CAD build for the part. Positions are in the model's coordinates, mm. Coordinates: 2 decimals unless noted, no trailing zeros. Write each loop counter-clockwise with the first axis right and the second up, starting at its lowest first coordinate (ties: lowest second). Pieces come first, ordered by that corner, then holes. Notation, with made-up numbers: (31, 73.5) - (65, 73.5) arc R15 ccw to (65, 99.5) - close; hole circle Ø4 at (69, 43.5). An arc over 180 degrees is marked (long way). One line per question, with ' | ' between items. Start each with the question number.
1. Two-plate mould, pull along Z, no slides. Class faces 1 (the flat face through (-33, 5, 10)), 2 (the cylindrical face through (-37.043, 2.465, 3.148)): +Z half, -Z half, draft (parallel to the pull), parting line (faces both ways), or undercut.
2. Flat gauge pins, fed straight in: P1, Ø4.5, axis at x = 27.21, z = -29.32, coming from the +Y side; P2, Ø6.5, axis at x = -39.89, z = 2.99, coming from the -Y side; P3, Ø1, axis at y = 0.5, z = -29.5, coming from the -X side; P4, Ø2, axis at y = 3.5, z = 12, coming from the +X side (3 decimals). Where does each tip first touch, or does it go through?
3. Band-saw the part on C-C, the plane z = -20. Write the cut outline in (x, y).
4. Band-saw the part on D-D, the plane y = 1.25. Give the number of separate pieces and of enclosed holes in the cut face, then the cut area to 3 significant figures.
5. Probe line 1 (X direction, y = 4, z = 0.5); line 2 (Z direction, x = -17, y = 2.95); line 3 (Z direction, x = 25, y = 1.3). List the from-to ranges inside material, lowest first.
6. Band-saw the part on A-A, the plane x = 0. Write the cut outline in (y, z).
7. Band-saw the part on B-B, the plane z = -46. Write the cut outline in (x, y).
from build123d import *

# Parameters (mm, degrees)
SKIZZE1_R                        = 50
SKIZZE1_R_2                      = 33.5
AUFSATZ_LINEAR_AUSTRAGEN1_DEPTH  = 5
F_3_2_3_2_DURCHMESSER_BOHRUNG2_D = 3.2
KREISMUSTER1_COUNT               = 7
F_5_6_5_6_DURCHMESSER_BOHRUNG2_D = 5.7
KREISMUSTER2_COUNT               = 21


with BuildPart() as part:
    # Skizze1 → Aufsatz-Linear austragen1 (new body)
    with BuildSketch(Plane(origin=(0, 0, 0), x_dir=(1, 0, 0), z_dir=(0, 1, 0))):
        with Locations(Location((0, 0, 0), (0, 0, 270))):
            Circle(SKIZZE1_R)
        with Locations(Location((0, 0, 0), (0, 0, 270))):
            Circle(SKIZZE1_R_2, mode=Mode.SUBTRACT)
    extrude(amount=AUFSATZ_LINEAR_AUSTRAGEN1_DEPTH)

    # Ø3.2 (3.2) Durchmesser Bohrung2 (through all)
    with Locations(Plane(origin=(0, 5, 0), x_dir=(1, 0, 0), z_dir=(0, 1, 0))):
        with Locations((0, 46)):
            f_3_2_3_2_durchmesser_bohrung2 = Hole(F_3_2_3_2_DURCHMESSER_BOHRUNG2_D / 2)

    # Kreismuster1: Ø3.2 (3.2) Durchmesser Bohrung2 ×7 about axis
    kreismuster1_axis = Axis((0, 0, 0), (0, 1, 0))
    for i in range(1, KREISMUSTER1_COUNT):
        add(f_3_2_3_2_durchmesser_bohrung2.rotate(kreismuster1_axis, i * 360 / KREISMUSTER1_COUNT), mode=Mode.SUBTRACT)

    # Ø5.6 (5.6) Durchmesser Bohrung2 (through all)
    with Locations(Plane(origin=(0, 5, 0), x_dir=(1, 0, 0), z_dir=(0, 1, 0))):
        with Locations((0, -40)):
            f_5_6_5_6_durchmesser_bohrung2 = Hole(F_5_6_5_6_DURCHMESSER_BOHRUNG2_D / 2)

    # Kreismuster2: Ø5.6 (5.6) Durchmesser Bohrung2 ×21 about axis
    kreismuster2_axis = Axis((0, 0, 0), (0, 1, 0))
    for i in range(1, KREISMUSTER2_COUNT):
        add(f_5_6_5_6_durchmesser_bohrung2.rotate(kreismuster2_axis, i * 360 / KREISMUSTER2_COUNT), mode=Mode.SUBTRACT)


solid = part.part
Filled in:
1) face 1: draft | face 2: undercut
2) P1: passes through | P2: stops at y = 0 | P3: stops at x = -40.73 | P4: stops at x = 48.775
3) outline: (-45.83, 0) - (-37.49, 0) - (-37.49, 5) - (-45.83, 5) - close; (-31.79, 0) - (-26.87, 0) - (-26.87, 5) - (-31.79, 5) - close; (26.87, 0) - (31.79, 0) - (31.79, 5) - (26.87, 5) - close; (37.49, 0) - (45.83, 0) - (45.83, 5) - (37.49, 5) - close
4) separate pieces: 1 | enclosed holes: 29 | area: 3,740 mm²
5) line 1: x = -50 to -41.28, -38.5 to -33.5, 33.5 to 38.5, 41.28 to 50 | line 2: z = -47.02 to -38.87, -33.21 to -28.87, 28.87 to 47.02 | line 3: z = -43.3 to -31.13, -27.52 to -22.3, 22.3 to 31.62, 34.48 to 43.3
6) outline: (0, -50) - (5, -50) - (5, -47.6) - (0, -47.6) - close; (0, -44.4) - (5, -44.4) - (5, -33.5) - (0, -33.5) - close; (0, 33.5) - (5, 33.5) - (5, 37.15) - (0, 37.15) - close; (0, 42.85) - (5, 42.85) - (5, 50) - (0, 50) - close
7) outline: (-19.6, 0) - (-1.6, 0) - (-1.6, 5) - (-19.6, 5) - close; (1.6, 0) - (19.6, 0) - (19.6, 5) - (1.6, 5) - close
